```python
from build123d import *

# Parameters (mm, degrees)
BOSS_EXTRUDE1_DEPTH = 12.7
SKETCH2_W           = 2.488429633
SKETCH2_H           = 2.032
CUT_EXTRUDE1_DEPTH  = 12.7


with BuildPart() as part:
    # Sketch1 → Boss-Extrude1 (new body)
    with BuildSketch(Plane(origin=(0, 0, 0), x_dir=(1, 0, 0), z_dir=(0, 1, 0))):
        with BuildLine():
            ThreePointArc((8.763, -3.175), (9.167603241, -4.582709081), (8.077288748, -3.60466872))
            Line((8.077288748, -3.60466872), (8.305859166, -3.715445814))
            ThreePointArc((8.305859166, -3.715445814), (9.032735494, -4.367472721), (8.763, -3.429))
            Line((8.763, -3.429), (1.27, -3.429))
            ThreePointArc((1.27, -3.429), (0.192369265, -2.982630735), (-0.254, -1.905))
            Line((-0.254, -1.905), (-0.254, 1.905))
            ThreePointArc((-0.254, 1.905), (0.192369265, 2.982630735), (1.27, 3.429))
            Line((1.27, 3.429), (8.763, 3.429))
            ThreePointArc((8.763, 3.429), (9.032735494, 4.367472721), (8.305859166, 3.715445814))
            Line((8.305859166, 3.715445814), (8.077288748, 3.60466872))
            ThreePointArc((8.077288748, 3.60466872), (9.167603241, 4.582709081), (8.763, 3.175))
            Line((8.763, 3.175), (1.27, 3.175))
            ThreePointArc((1.27, 3.175), (0.371974388, 2.803025612), (0, 1.905))
            Line((0, 1.905), (0, -1.905))
            ThreePointArc((0, -1.905), (0.371974388, -2.803025612), (1.27, -3.175))
            Line((1.27, -3.175), (8.763, -3.175))
        make_face()
    extrude(amount=BOSS_EXTRUDE1_DEPTH)

    # Sketch2 → Cut-Extrude1 (cut)
    with BuildSketch(Plane.ZY.offset(0.254)):
        with Locations((-4.673214816, 8.382)):
            Rectangle(SKETCH2_W, SKETCH2_H)
        with Locations((-4.673214816, 4.318)):
            Rectangle(SKETCH2_W, SKETCH2_H)
    cut_extrude1 = extrude(amount=-CUT_EXTRUDE1_DEPTH, mode=Mode.SUBTRACT)

    # Mirror1: Cut-Extrude1 across plane
    add(cut_extrude1.mirror(Plane(origin=(0, 0, 0), x_dir=(1, 0, 0), z_dir=(0, 0, -1))), mode=Mode.SUBTRACT)


solid = part.part
```
Read the model definition and answer for the solid it produces. Units are mm, in the model's axes. A direction names the side the tool comes from. Round coordinates to 2 decimals unless told otherwise and drop trailing zeros. Write each loop counter-clockwise with the first axis right and the second up, starting at its lowest first coordinate (ties: lowest second). Pieces come first, ordered by that corner, then holes. Notation, with made-up numbers: (-36.5, -25) - (21.5, -25) arc R24 ccw to (21.5, -4) - close; hole circle Ø10 at (23.25, 39). An arc over 180 degrees is marked (long way). One line per item, written item: value.
Q1. Find section B-B (y = 6). Determine the outline of the cut face in (x, z) (3 decimals).
The answers:
outline: (-0.254, -1.905) arc R1.524 ccw to (1.27, -3.429) - (8.763, -3.429) arc R0.508 cw (long way) to (8.306, -3.715) - (8.077, -3.605) arc R0.762 ccw (long way) to (8.763, -3.175) - (1.27, -3.175) arc R1.27 cw to (0, -1.905) - (0, 1.905) arc R1.27 cw to (1.27, 3.175) - (8.763, 3.175) arc R0.762 ccw (long way) to (8.077, 3.605) - (8.306, 3.715) arc R0.508 cw (long way) to (8.763, 3.429) - (1.27, 3.429) arc R1.524 ccw to (-0.254, 1.905) - close
Q2. Find section D-D (z = -1). Determine the outline of the cut face in (x, y), and give its area (3 significant figures).
The answers:
outline: (-0.25, 0) - (0, 0) - (0, 12.7) - (-0.25, 12.7) - close
area: 3.23 mm2
Q3. Find section A-A (x = 5.75). Determine the outline of the cut face in (y, z) (3 decimals), and give its area (3 significant figures).
The answers:
outline: (0, -3.429) - (12.7, -3.429) - (12.7, -3.175) - (0, -3.175) - close; (0, 3.175) - (12.7, 3.175) - (12.7, 3.429) - (0, 3.429) - close
area: 6.45 mm2
Q4. For a pull along Z with two mould halves and no side action, classify faces 1 (the cylindrical face through (0.36, 6.26, 2.79)), 2 (the cylindrical face through (0.18, 6.26, -2.97)), 3 (the flat face through (-0.254, 6, 0)) as pulls with the +Z half, pulls with the -Z half, needs draft (parallel to the pull), parting line crosses it, or undercut.
The answers:
face 1: undercut
face 2: pulls with the -Z half
face 3: needs draft
Q5. Each of these flat-tipped pins is pushed along its axis until it touches: P1, Ø4, axis at x = 5.5, y = 9.5, coming from the +Z side; P2, Ø2, axis at x = 5.5, y = 7.5, coming from the -Z side; P3, Ø3, axis at y = 7.5, z = 0.5, coming from the +X side. Where does it stop, or does it pass through?
The answers:
P1: stops at z = 3.43
P2: stops at z = -3.43
P3: stops at x = 0
Q6. Find section C-C (z = -4). Determine the outline of the cut face in (x, y), and give its area (3 significant figures).
The answers:
outline: (8, 0) - (8.26, 0) - (8.26, 3.3) - (8, 3.3) - close; (8, 5.33) - (8.26, 5.33) - (8.26, 7.37) - (8, 7.37) - close; (8, 9.4) - (8.26, 9.4) - (8.26, 12.7) - (8, 12.7) - close; (9.27, 0) - (9.52, 0) - (9.52, 3.3) - (9.27, 3.3) - close; (9.27, 5.33) - (9.52, 5.33) - (9.52, 7.37) - (9.27, 7.37) - close; (9.27, 9.4) - (9.52, 9.4) - (9.52, 12.7) - (9.27, 12.7) - close
area: 4.41 mm2
Q7. Straight lines are drawn through the part: line 1 (Z direction, x = 5.75, y = 11.5) (3 decimals); line 2 (X direction, y = 3.25, z = 1.5); line 3 (Z direction, x = 0.5, y = 8). For each, find the intervals that lie inside material, in ascending order. Write a range as from..to.
The answers:
line 1: z = -3.429..-3.175, 3.175..3.429
line 2: x = -0.25..0
line 3: z = -3.22..-2.91, 2.91..3.22
Q8. Which of the six approach directions +Z, -Z, +X, -X, +Y, -Y give full straight-line access (tool end or side, diameter ignored) to faces 4 (the cylindrical face through (9.017, 1.628, 4.377)), 5 (the flat face through (5, 6, 3.175))?
The answers:
face 4: +Y, -Y
face 5: +X, +Y, -Y
